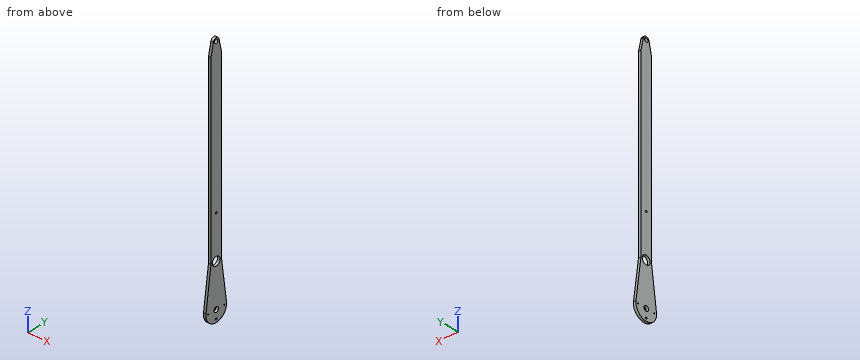
from build123d import *

# Parameters (mm, degrees)
SKETCH1_R             = 6.35
SKETCH1_R_2           = 11.1125
SKETCH1_R_3           = 4.7625
BOSS_EXTRUDE1_DEPTH   = 3.175
M3X0_5_TAPPED_HOLE1_D = 2.5
M4_CLEARANCE_HOLE1_D  = 4.5


with BuildPart() as part:
    # Sketch1 → Boss-Extrude1 (new, symmetric)
    with BuildSketch(Plane(origin=(0, 0, 0), x_dir=(0, 0, -1), z_dir=(1, 0, 0))):
        with BuildLine():
            Line((-470, 15), (-501.760727799, 8.072716015))
            ThreePointArc((-501.760727799, 8.072716015), (-508.2625, 0), (-501.760727799, -8.072716015))
            Line((-501.760727799, -8.072716015), (-470, -15))
            Line((-470, -15), (0, -15))
            Line((0, -15), (106.075609583, -29.237803609))
            ThreePointArc((106.075609583, -29.237803609), (139.5, 0), (106.075609583, 29.237803609))
            Line((106.075609583, 29.237803609), (0, 15))
            Line((0, 15), (-470, 15))
        make_face()
        with Locations((110, 0)):
            Circle(SKETCH1_R, mode=Mode.SUBTRACT)
        Circle(SKETCH1_R_2, mode=Mode.SUBTRACT)
        with Locations((-500, 0)):
            Circle(SKETCH1_R_3, mode=Mode.SUBTRACT)
    extrude(amount=BOSS_EXTRUDE1_DEPTH, both=True)

    # M3x0.5 Tapped Hole1 (through all)
    with Locations(Plane(origin=(3.175, 0, 0), x_dir=(0, 0, -1), z_dir=(1, 0, 0))):
        with Locations((110, 23.015), (110, 0), (110, -23.015)):
            Hole(M3X0_5_TAPPED_HOLE1_D / 2)

    # M4 Clearance Hole1 (through all)
    with Locations(Plane(origin=(3.175, 0, 0), x_dir=(0, 0, -1), z_dir=(1, 0, 0))):
        with Locations((131.5, 0), (-110, 0)):
            Hole(M4_CLEARANCE_HOLE1_D / 2)


solid = part.part
Part model, mm, in its own coordinate system. Round coordinates to 2 decimals unless told otherwise and drop trailing zeros. Loops run counter-clockwise (first coordinate to the right, second up) from the corner with the lowest first, then second, coordinate; pieces in that order, holes last. Notation, with made-up numbers: (-38.75, -33) - (4.25, -33) arc R18 ccw to (4.25, -23) - close; hole circle Ø2 at (62.25, 36). An arc over 180 degrees is marked (long way). Answer as a JSON object with one key per item and string values.
Item 1: Band-saw the part on B-B on z = 29. List the corners of the cut face in (x, y) (3 decimals).
Output:
{"outline": "(-3.175, -15) - (3.175, -15) - (3.175, 15) - (-3.175, 15) - close"}
Item 2: Pin check, flat tips, straight feed: pin 1 (3 mm diameter, centred on x = -2.5, z = 389, fed in from -Y); pin 2 (1.5 mm diameter, centred on x = 1.5, y = 1, fed in from +Z); pin 3 (1.5 mm diameter, centred on y = 23.015, z = -110, fed in from +X). Stop position of each tip, or through.
Output:
{"pin 1": "y = -15", "pin 2": "z = 508.26", "pin 3": "through"}
Item 3: Band-saw the part on A-A on x = 1.5. State how many separate pieces and enclosed holes the cut face has, plus the area to 3 significant figures.
Output:
{"separate pieces": "1", "enclosed holes": "7", "area": "20,600 mm2"}
Item 4: Wall check: L1, parallel to Y at x = 1, z = -110 (3 decimals); L2, parallel to Z at x = -0.5, y = 0.5; L3, parallel to Z at x = -1.25, y = 3.5. Give the ranges that are in metal, low to high.
Output:
{"L1": "-29.5 to -24.265, -21.765 to -6.35, 6.35 to 21.765, 24.265 to 29.5", "L2": "-139.5 to -133.69, -129.31 to -116.33, -103.67 to -11.1, 11.1 to 107.81, 112.19 to 495.26, 504.74 to 508.25", "L3": "-139.29 to -115.3, -104.7 to -10.55, 10.55 to 496.77, 503.23 to 507.48"}
